Could you check a few things on this model? Use its own coordinates, in mm. Give positions to 0.01 mm unless a question says otherwise; leave off trailing zeros. Write each loop counter-clockwise with the first axis right and the second up, starting at its lowest first coordinate (ties: lowest second). Pieces come first, ordered by that corner, then holes. Notation, with made-up numbers: M 73,35 L 90,35 A28 cw 90,67 Z; hole C 58,83 d6. An arc over 180 degrees is marked long. Write each question's results on one line, items separated by ' | '. Start each with the question number.
from build123d import *

# Parameters (mm, degrees)
SKETCH1_W               = 80
SKETCH1_H               = 75
BOSS_EXTRUDE1_DEPTH     = 30
CUT_EXTRUDE3_DEPTH      = 30
CUT_EXTRUDE4_DEPTH      = 46
CUT_EXTRUDE4_DEPTH_BACK = 53


with BuildPart() as part:
    # Sketch1 → Boss-Extrude1 (new body)
    with BuildSketch(Plane(origin=(0, 0, 0), x_dir=(1, 0, 0), z_dir=(0, 1, 0))):
        with Locations((-35.837742504, -33.866843034)):
            Rectangle(SKETCH1_W, SKETCH1_H)
    extrude(amount=BOSS_EXTRUDE1_DEPTH)

    # Sketch6 → Cut-Extrude3 (cut)
    with BuildSketch(Plane(origin=(0, 30, 0), x_dir=(1, 0, 0), z_dir=(0, 1, 0))):
        with BuildLine():
            Line((-71.375833468, 3.633156966), (-108.820806999, 13.42149107))
            Line((-108.820806999, 13.42149107), (-125.584570218, -100.370099881))
            Line((-125.584570218, -100.370099881), (-10.920024304, -107.668906036))
            Line((-10.920024304, -107.668906036), (16.042240316, -75.531910929))
            Line((16.042240316, -75.531910929), (16.042240316, -32.24724925))
            Line((16.042240316, -32.24724925), (13.170421527, 8.096312294))
            Line((13.170421527, 8.096312294), (0.934093701, 3.633156966))
            ThreePointArc((0.934093701, 3.633156966), (3.278926231, -13.213255463), (4.162257496, -30.199119503))
            Line((4.162257496, -30.199119503), (-25.2116582, -30.199119503))
            Line((-25.2116582, -30.199119503), (-25.2116582, -71.366843034))
            Line((-25.2116582, -71.366843034), (-65.403764634, -71.366843034))
            ThreePointArc((-65.403764634, -71.366843034), (-68.14206018, -67.273150859), (-70.111731546, -62.759064813))
            ThreePointArc((-70.111731546, -62.759064813), (-75.817600676, -29.659558964), (-71.375833468, 3.633156966))
        make_face()
    extrude(amount=-CUT_EXTRUDE3_DEPTH, mode=Mode.SUBTRACT)

    # Sketch7 → Cut-Extrude4 (cut, two sides: drawn at the far end of the back side and taken through both)
    with BuildSketch(Plane(origin=(-25.2116582, 0, 0), x_dir=(0, 0, -1), z_dir=(1, 0, 0)).offset(-CUT_EXTRUDE4_DEPTH_BACK)):
        with BuildLine():
            Line((3.633156966, 4.41216157), (25.866454997, 63.394578765))
            Line((25.866454997, 63.394578765), (-68.187233435, 84.334388308))
            Line((-68.187233435, 84.334388308), (-84.699418689, 46.854351889))
            Line((-84.699418689, 46.854351889), (-91.169251259, 32.168860137))
            Line((-91.169251259, 32.168860137), (-79.899921895, -15.478262788))
            Line((-79.899921895, -15.478262788), (10.487341479, -37.061233348))
            Line((10.487341479, -37.061233348), (3.633156966, 2.319452889))
            ThreePointArc((3.633156966, 2.319452889), (-33.958413843, 0.084026639), (-71.366843034, 4.41216157))
            Line((-71.366843034, 4.41216157), (-77.914841613, 5.869986833))
            Line((-77.914841613, 5.869986833), (-71.366843034, 6.525778375))
            ThreePointArc((-71.366843034, 6.525778375), (-33.960238488, 2.154907065), (3.633156966, 4.41216157))
        make_face()
    extrude(amount=CUT_EXTRUDE4_DEPTH + CUT_EXTRUDE4_DEPTH_BACK, mode=Mode.SUBTRACT)


solid = part.part
Q1. If we mould it in two halves opening along Z, with no side actions, what happens to faces 1 (the face through (-75.808, 1.401, 30.131)), 2 (the face through (-25.212, 3, 51)), 3 (the face through (-10, 1, 30.199)), 4 (the face through (-45.288, 2.078, 26.109))? For each: pulls with the +Z half, pulls with the -Z half, needs draft (parallel to the pull), parting line crosses it, or undercut.
Q2. I'm going to push flat-ended pins straight in: P1, Ø1, axis at x = -47.5, z = 20.5, coming from the -Y side; P2, Ø12, axis at x = -25, z = 25, coming from the +Y side; P3, Ø2.5, axis at x = -6.5, y = 1.5, coming from the +Z side. Where does each tip first touch, or does it pass through?
Q3. If we section it at A-A (x = -40.5): Please give me the cut outline in (y, z).
Q4. Please list where these lines run through material, in increasing order: line 1 (X direction, y = 3, z = 57.5); line 2 (X direction, y = 3, z = 56); line 3 (Y direction, x = -37, z = 13.5). Write a range as [from, to].
Q5. If we section it at B-B (z = 22): Please give me the cut outline in (x, y).
Determined:
1) face 1: parting line crosses it | face 2: needs draft | face 3: pulls with the +Z half | face 4: undercut
2) P1: stops at y = 0.11 | P2: stops at y = 2.26 | P3: stops at z = 30.2
3) outline: M 2.32,-3.63 L 4.41,-3.63 A213.91 cw 6.53,71.37 L 4.41,71.37 A215.98 ccw Z
4) line 1: x = [-71.72, -25.21] | line 2: x = [-72.13, -25.21] | line 3: y = [0.48, 2.56]
5) outline: M -75.7,0.08 L 3.92,0.08 L 3.92,2.15 L -75.7,2.15 Z
